Could you check a few things on this model? Use its own coordinates, in mm. A direction names the side the tool comes from. Give positions to 0.01 mm unless a question says otherwise; leave off trailing zeros. Loops run counter-clockwise (first coordinate to the right, second up) from the corner with the lowest first, then second, coordinate; pieces in that order, holes last. Notation, with made-up numbers: (-5, -30) -> (31, -30) arc R16 cw to (31, -21) -> close; hole circle Ø2 at (66.25, 86.5). An arc over 180 degrees is marked (long way). Write item = value, one per line. Start each with the question number.
1) On a 3-axis mill with a long thin cutter (end or side, diameter ignored), from which of +Z, -Z, +X, -X, +Y, -Y can I reach the whole of each face in a straight line? I mean faces 4 (the face through (40, -5.75, 14)), 5 (the face through (-20, 38, 33)), 6 (the face through (-12.928, 39.862, 35.028)), 7 (the face through (38, 27.75, 20)). Say none if no direction works.
2) I want a section at B-B (x = -20). List the corners of the cut face in (y, z) for me.
3) I want a section at D-D (x = 21.25). Count the separate pieces of the cut face and the enclosed holes in it, and give its area (3 significant figures).
4) I'm going to push flat-ended pins straight in: pin 1 Ø5 at (x, y) = (-2, 18) entering from +Z; pin 2 Ø6 at (x, z) = (-28, 13.5) entering from +Y; pin 3 Ø4 at (x, y) = (-32.25, -10.75) entering from +Z. Where does each tip first touch, or does it pass through?
5) If we mould it in two halves opening along Z, with no side actions, what happens to faces 1 (the face through (-18.79, 43.647, 35.028)), 2 (the face through (43, 24.75, 14)), 3 (the face through (2, 0, 0))? For each: +Z half, -Z half, draft (parallel to the pull), parting line (faces both ways), or undercut.
6) I want a section at C-C (z = 19). List the corners of the cut face in (x, y) for me, and give its area (3 significant figures).
7) I need wall thicknesses on probe 1 along Y at (x, z) = (-20, 35); probe 2 along Y at (x, z) = (21.25, 1.9); probe 3 along Y at (x, z) = (-20.5, 23.5). Which ranges of each line are inside material? Lowest first, please. Write a range as from..to.
8) I want a section at A-A (y = 17). List the corners of the cut face in (x, z) for me.
from build123d import *

# Parameters (mm, degrees)
SKETCH_1_W          = 83.5
SKETCH_1_H          = 63.5
SKETCH_1_R          = 1.5
EXTRUDE_1_DEPTH     = 3
EXTRUDE_START       = 3
EXTRUDE_2_DEPTH     = 15
EXTRUDE_START_2     = 18
EXTRUDE_3_DEPTH     = 19
SKETCH_1_5_W        = 3
SKETCH_1_5_H        = 9
EXTRUDE_6_DEPTH     = 4
SKETCH_6_R          = 2.25
EXTRUDE_7_DEPTH     = 4
SKETCH_7_W          = 3
SKETCH_7_H          = 9
SKETCH_7_W_2        = 9
SKETCH_7_H_2        = 12
EXTRUDE_8_DEPTH     = 16
SKETCH_8_W          = 10
SKETCH_8_H          = 2
CUT_EXTRUDE_1_DEPTH = 34
SKETCH_9_R          = 2.5
SKETCH_9_R_2        = 1.5
EXTRUDE_17_DEPTH    = 3


with BuildPart() as part:
    # 草图1 → 凸台-拉伸1 (new body)
    with BuildSketch(Plane.XY):
        with Locations((2.5, 0)):
            Rectangle(SKETCH_1_W, SKETCH_1_H)
        with Locations((21.25, -24.75)):
            Circle(SKETCH_1_R, mode=Mode.SUBTRACT)
        with Locations((21.25, 24.75)):
            Circle(SKETCH_1_R, mode=Mode.SUBTRACT)
        with Locations((-32.25, -10.75)):
            Circle(SKETCH_1_R, mode=Mode.SUBTRACT)
    extrude(amount=EXTRUDE_1_DEPTH)

    # 草图1<3> → 凸台-拉伸2 (add)
    with BuildSketch(Plane.XY.offset(EXTRUDE_START)):
        Polygon((35.25, -27.75), (-35.25, -27.75), (-35.25, 27.75), (41.25, 27.75), (41.25, 24.75), (44.25, 24.75), (44.25, 31.75), (-39.25, 31.75), (-39.25, -31.75), (44.25, -31.75), (44.25, -17.75), (35.25, -17.75), align=None)
        Polygon((35.25, 12.75), (35.25, -5.75), (44.25, -5.75), (44.25, 15.75), (41.25, 15.75), (41.25, 12.75), align=None)
    extrude(amount=EXTRUDE_2_DEPTH)

    # 草图1<4> → 凸台-拉伸3 (add)
    with BuildSketch(Plane.XY.offset(EXTRUDE_START_2)):
        Polygon((35.25, -27.75), (-35.25, -27.75), (-35.25, 27.75), (41.25, 27.75), (41.25, 24.75), (44.25, 24.75), (44.25, 31.75), (-39.25, 31.75), (-39.25, -31.75), (44.25, -31.75), (44.25, -17.75), (35.25, -17.75), align=None)
        Polygon((35.25, 12.75), (35.25, -5.75), (44.25, -5.75), (44.25, 15.75), (41.25, 15.75), (41.25, 12.75), align=None)
    extrude(amount=EXTRUDE_3_DEPTH)

    # 草图1<5> → 凸台-拉伸6 (add)
    with BuildSketch(Plane.XY.offset(EXTRUDE_START)):
        with Locations((42.75, 20.25)):
            Rectangle(SKETCH_1_5_W, SKETCH_1_5_H)
        Polygon((35.25, -5.75), (35.25, -17.75), (41.25, -17.75), (44.25, -17.75), (44.25, -5.75), (41.25, -5.75), align=None)
    extrude(amount=EXTRUDE_6_DEPTH)

    # 草图6 → 凸台-拉伸7 (add)
    # profile 1 of 2: a face of its own
    with BuildSketch(Plane.XY.offset(37)):
        Polygon((30.024768978, 31.75), (24.201245229, 47.75), (15.798754771, 47.75), (9.975231022, 31.75), align=None)
        with Locations((20, 41.75)):
            Circle(SKETCH_6_R, mode=Mode.SUBTRACT)
    # profile 2 of 2: a face of its own
    with BuildSketch(Plane.XY.offset(37)):
        Polygon((-24.201245229, 47.75), (-15.798754771, 47.75), (-9.975231022, 31.75), (-30.024768978, 31.75), align=None)
        with Locations((-20, 41.75)):
            Circle(SKETCH_6_R, mode=Mode.SUBTRACT)
    extrude(amount=-EXTRUDE_7_DEPTH)

    # 草图7 → 凸台-拉伸8 (add)
    with BuildSketch(Plane.XY.offset(37)):
        with Locations((42.75, 20.25)):
            Rectangle(SKETCH_7_W, SKETCH_7_H)
        with Locations((39.75, -11.75)):
            Rectangle(SKETCH_7_W_2, SKETCH_7_H_2)
    extrude(amount=-EXTRUDE_8_DEPTH)

    # 草图8 → 切除-拉伸1 (cut)
    with BuildSketch(Plane.XY.offset(37)):
        with Locations((30.25, 28.75)):
            Rectangle(SKETCH_8_W, SKETCH_8_H)
    extrude(amount=-CUT_EXTRUDE_1_DEPTH, mode=Mode.SUBTRACT)

    # 草图9 → 凸台-拉伸17 (add)
    # profile 1 of 3: a face of its own
    with BuildSketch(Plane.XY.offset(3)):
        with Locations((-32.25, -10.75)):
            Circle(SKETCH_9_R)
        with Locations((-32.25, -10.75)):
            Circle(SKETCH_9_R_2, mode=Mode.SUBTRACT)
    # profile 2 of 3: a face of its own
    with BuildSketch(Plane.XY.offset(3)):
        with Locations((21.25, 24.75)):
            Circle(SKETCH_9_R)
        with Locations((21.25, 24.75)):
            Circle(SKETCH_9_R_2, mode=Mode.SUBTRACT)
    # profile 3 of 3: a face of its own
    with BuildSketch(Plane.XY.offset(3)):
        with Locations((21.25, -24.75)):
            Circle(SKETCH_9_R)
        with Locations((21.25, -24.75)):
            Circle(SKETCH_9_R_2, mode=Mode.SUBTRACT)
    extrude(amount=EXTRUDE_17_DEPTH)


solid = part.part
Answer list:
q1.face_4 = +X
q1.face_5 = -Z, +X, -X, +Y
q1.face_6 = +Z, -Z, +Y
q1.face_7 = +Z
q2.outline = (-31.75, 0) -> (31.75, 0) -> (31.75, 33) -> (39.5, 33) -> (39.5, 37) -> (27.75, 37) -> (27.75, 3) -> (-27.75, 3) -> (-27.75, 37) -> (-31.75, 37) -> close; (44, 33) -> (47.75, 33) -> (47.75, 37) -> (44, 37) -> close
q3.separate_pieces = 4
q3.enclosed_holes = 0
q3.area = 506 mm^2
q4.pin_1 = 3
q4.pin_2 = 31.75
q4.pin_3 = 6
q5.face_1 = draft
q5.face_2 = undercut
q5.face_3 = -Z half
q6.outline = (-39.25, -31.75) -> (44.25, -31.75) -> (44.25, -17.75) -> (35.25, -17.75) -> (35.25, -27.75) -> (-35.25, -27.75) -> (-35.25, 27.75) -> (25.25, 27.75) -> (25.25, 29.75) -> (35.25, 29.75) -> (35.25, 27.75) -> (41.25, 27.75) -> (41.25, 24.75) -> (44.25, 24.75) -> (44.25, 31.75) -> (-39.25, 31.75) -> close; (35.25, -5.75) -> (44.25, -5.75) -> (44.25, 15.75) -> (41.25, 15.75) -> (41.25, 12.75) -> (35.25, 12.75) -> close
q6.area = 1,140 mm^2
q7.probe_1 = -31.75..-27.75, 27.75..39.5, 44..47.75
q7.probe_2 = -31.75..-26.25, -23.25..23.25, 26.25..31.75
q7.probe_3 = -31.75..-27.75, 27.75..31.75
q8.outline = (-39.25, 0) -> (44.25, 0) -> (44.25, 7) -> (41.25, 7) -> (41.25, 3) -> (-35.25, 3) -> (-35.25, 37) -> (-39.25, 37) -> close; (41.25, 21) -> (44.25, 21) -> (44.25, 37) -> (41.25, 37) -> close
